Input: part model. Units: mm. Frame: model coordinates. A direction names the side the tool comes from. Give positions to 0.01 mm unless a question says otherwise; leave off trailing zeros. Order: outer loops, then holes, each group sorted by start corner. A loop starts at its lowest first (then second) coordinate and runs counter-clockwise, first axis right, second up. Notation, with made-up numbers: M -4.75,74 L 48.25,74 A20 ccw 48.25,95 Z; hole C -37.75,57 d6. An arc over 180 degrees is marked long. Use a Markdown table: item, result.
from build123d import *

# Parameters (mm, degrees)
SKETCH1_R           = 44.75
BOSS_EXTRUDE1_DEPTH = 4
SKETCH2_R           = 47.75
BOSS_EXTRUDE2_DEPTH = 4


with BuildPart() as part:
    # Sketch1 → Boss-Extrude1 (new body)
    with BuildSketch(Plane.XY):
        Circle(SKETCH1_R)
    extrude(amount=BOSS_EXTRUDE1_DEPTH)

    # Sketch2 → Boss-Extrude2 (add)
    with BuildSketch(Plane.XY.offset(4)):
        Circle(SKETCH2_R)
    extrude(amount=BOSS_EXTRUDE2_DEPTH)

    # Sketch3 → Cut-Revolve1 (revolve, cut)
    with BuildSketch(Plane(origin=(0, 0, 0), x_dir=(0, 0, -1), z_dir=(1, 0, 0))):
        with BuildLine():
            Line((-4, 47.75), (-4, 44.75))
            add(Edge.make_bspline(
                [(-4, 44.75), (-5.51655106, 47.70034682), (-8, 47.75)],
                knots=[0, 0, 0, 0.96689788, 0.96689788, 0.96689788], degree=2))
            Line((-8, 47.75), (-4, 47.75))
        make_face()
    revolve(axis=Axis((0, 0, 14.618090142), (0, 0, -1)), mode=Mode.SUBTRACT)

    # Sketch4 → Cut-Revolve3 (revolve, cut)
    with BuildSketch(Plane(origin=(0, 0, 0), x_dir=(0, 0, -1), z_dir=(1, 0, 0))):
        with BuildLine():
            Line((-4.667863656, 44.75), (-4.217612647, 44.75))
            Line((-4.217612647, 44.75), (-4.442738152, 0))
            Line((-4.442738152, 0), (-8, 0))
            Line((-8, 0), (-8, 47.272851402))
            add(Edge.make_bspline(
                [(-8, 47.272851402), (-5.020669257, 46.35865801), (-4.667863656, 44.75)],
                knots=[0, 0, 0, 0.52721511, 0.52721511, 0.52721511], degree=2))
        make_face()
    revolve(axis=Axis((0, 0, 4.442738152), (0, 0, 1)), mode=Mode.SUBTRACT)


solid = part.part
1) Reachability of faces 1 (the face through (20.65, -39.7, 1.97)), 2 (the face through (2.12, -0.47, 4.43)), 3 (the face through (-46.2, 10.8, 8)) from +Z, -Z, +X, -X, +Y, -Y: full face, straight path, thin tool, end or side. Return the list, or none.
Response values:
| item | result |
|---|---|
| face 1 | -Z |
| face 2 | +Z |
| face 3 | +Z, +X, -X, +Y, -Y |
2) First-contact query: pin 1 Ø2 at (x, y) = (10.5, -11.5) entering from +Z; pin 2 Ø1.5 at (x, z) = (30.5, 4) entering from -Y. Flat tips, straight axial feed; report the tip coordinate or a pass-through.
Response values:
| item | result |
|---|---|
| pin 1 | stops at z = 4.37 |
| pin 2 | stops at y = -34.53 |
3) Cut plane A-A on z = 2.5. Return loops of the section in (x, y).
Response values:
| item | result |
|---|---|
| outline | C 0,0 d89.5 |
4) Material intervals for line 1 (Z direction, x = -39.5, y = 12); line 2 (X direction, y = -24, z = 7.5); line 3 (X direction, y = 0, z = 4.5), sorted ascending. Write a range as from..to.
Response values:
| item | result |
|---|---|
| line 1 | z = 0..4.24 |
| line 2 | x = -41.23..-40.54, 40.54..41.23 |
| line 3 | x = -45.6..-44.75, 44.75..45.6 |
